from build123d import *

# Parameters (mm, degrees)
CHANFREIN1_SIZE                    = 0.5
CHANFREIN2_SIZE                    = 0.2
ESQUISSE2_R                        = 1.5
TROU_DE_FIXATION_DU_MOTEUR_DEPTH   = 36.860842154
R_P_TITION_DES_3_TROUS_COUNT       = 3
ESQUISSE3_R                        = 2.25
TROU_DE_FIXATION_DE_LA_BRIDE_DEPTH = 36.860842154
R_P_TITION_DES_4_TROUS_COUNT       = 4


with BuildPart() as part:
    # Esquisse1 → Base-R_volution (revolve)
    with BuildSketch(Plane.XY, mode=Mode.PRIVATE) as base_r_volution_sk:
        Polygon((-3, 3.25), (-3, 25), (0, 25), (0, 14.5), (3, 14.5), (3, 3.25), align=None)
    revolve(base_r_volution_sk.sketch.rotate(Axis((-30.73022942, 0, 0), (1, 0, 0)), 90), axis=Axis((-30.73022942, 0, 0), (1, 0, 0)))

    # Chanfrein1
    chanfrein1_edges = [part.edges().sort_by_distance(p)[0] for p in [
        (3, 0, -14.5),
    ]]
    chamfer(chanfrein1_edges, length=CHANFREIN1_SIZE)

    # Chanfrein2
    chanfrein2_edges = [part.edges().sort_by_distance(p)[0] for p in [
        (-3, 0, -25),
        (0, 0, -25),
    ]]
    chamfer(chanfrein2_edges, length=CHANFREIN2_SIZE)

    # Esquisse2 → Trou de fixation du moteur (cut, through all)
    with BuildSketch(Plane(origin=(3, 0, 0), x_dir=(0, 0, -1), z_dir=(1, 0, 0))):
        with Locations((-8.227241336, 4.75)):
            Circle(ESQUISSE2_R)
    trou_de_fixation_du_moteur = extrude(amount=-TROU_DE_FIXATION_DU_MOTEUR_DEPTH, mode=Mode.SUBTRACT)

    # R_p_tition des 3 trous: Trou de fixation du moteur ×3 about axis
    r_p_tition_des_3_trous_axis = Axis((0, 0, 0), (1, 0, 0))
    for i in range(1, R_P_TITION_DES_3_TROUS_COUNT):
        add(trou_de_fixation_du_moteur.rotate(r_p_tition_des_3_trous_axis, i * 360 / R_P_TITION_DES_3_TROUS_COUNT), mode=Mode.SUBTRACT)

    # Esquisse3 → Trou de fixation de la bride (cut, through all)
    with BuildSketch(Plane.ZY.offset(3)):
        with Locations((0, 21.5)):
            Circle(ESQUISSE3_R)
    trou_de_fixation_de_la_bride = extrude(amount=-TROU_DE_FIXATION_DE_LA_BRIDE_DEPTH, mode=Mode.SUBTRACT)

    # R_p_tition des 4 trous: Trou de fixation de la bride ×4 about axis
    r_p_tition_des_4_trous_axis = Axis((0, 0, 0), (1, 0, 0))
    for i in range(1, R_P_TITION_DES_4_TROUS_COUNT):
        add(trou_de_fixation_de_la_bride.rotate(r_p_tition_des_4_trous_axis, i * 360 / R_P_TITION_DES_4_TROUS_COUNT), mode=Mode.SUBTRACT)


solid = part.part
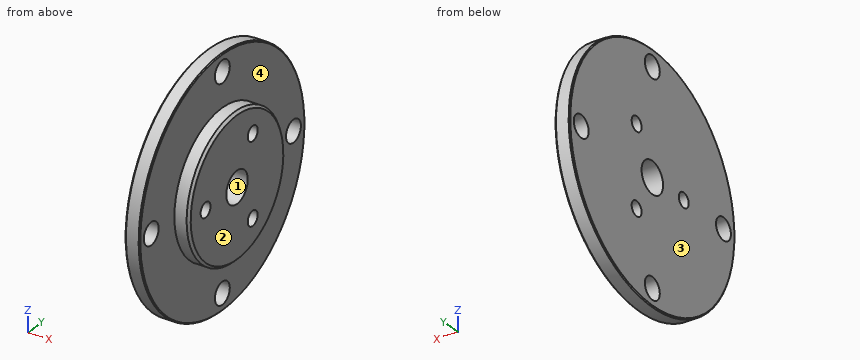
Check sheet for the modelled part. Datum: model origin and axes. Units: mm. Face numbers are marked on the shaded views. A direction names the side the tool comes from. Round coordinates to 2 decimals unless told otherwise and drop trailing zeros. Write each loop counter-clockwise with the first axis right and the second up, starting at its lowest first coordinate (ties: lowest second). Pieces come first, ordered by that corner, then holes. Notation, with made-up numbers: (34.5, 33) - (78.5, 33) arc R18 cw to (78.5, 68) - close; hole circle Ø4 at (-21, 83). An arc over 180 degrees is marked (long way). Return JSON: item names as keys, results as strings.
Q1. Cross-section at A-A (y = 0). Record the boundary of the cut face in (x, z).
Returned:
{"outline": "(-3, -24.8) - (-2.8, -25) - (-0.2, -25) - (0, -24.8) - (0, -23.75) - (-3, -23.75) - close; (-3, -19.25) - (0, -19.25) - (0, -14.5) - (2.5, -14.5) - (3, -14) - (3, -3.25) - (-3, -3.25) - close; (-3, 3.25) - (3, 3.25) - (3, 14) - (2.5, 14.5) - (0, 14.5) - (0, 19.25) - (-3, 19.25) - close; (-3, 23.75) - (0, 23.75) - (0, 24.8) - (-0.2, 25) - (-2.8, 25) - (-3, 24.8) - close"}
Q2. Access from +Z, -Z, +X, -X, +Y, -Y to the whole of each face (thin tool, end or side, straight path). Record for the marked faces 3 and 4.
Returned:
{"face 3": "+Z, -Z, -X, +Y, -Y", "face 4": "+X"}
Q3. Depth check by flat-ended pin: P1, Ø7, axis at y = 0, z = 21.5, coming from the +X side; P2, Ø1, axis at x = -1.5, z = -7.5, coming from the +Y side. Enter the tip coordinate at first touch or a pass-through.
Returned:
{"P1": "stops at x = 0", "P2": "stops at y = 24"}
Q4. Cross-section at B-B (x = 1.45). Record the boundary of the cut face in (y, z), then the cut area to 3 significant figures.
Returned:
{"outline": "circle Ø29 at (0, 0); hole circle Ø3 at (-9.5, 0); hole circle Ø6.5 at (0, 0); hole circle Ø3 at (4.75, -8.23); hole circle Ø3 at (4.75, 8.23)", "area": "606 mm²"}
Q5. Scan lines: L1, parallel to Y at x = 0.15, z = 0; L2, parallel to Y at x = -0.65, z = 0; L3, parallel to X at y = 20.5, z = -6. Record each from-to range of solid material in increasing order. Write a range as from..to.
Returned:
{"L1": "y = -14.5..-11, -8..-3.25, 3.25..14.5", "L2": "y = -25..-23.75, -19.25..-11, -8..-3.25, 3.25..19.25, 23.75..25", "L3": "x = -3..0"}
Q6. Draft check along Z on the marked faces 1 and 2. Enter one of: released by +Z, released by -Z, zero draft, split by the parting line, or undercut.
Returned:
{"face 1": "undercut", "face 2": "zero draft"}
